from build123d import *

# Parameters (mm, degrees)
SALIENTE_EXTRUIR1_DEPTH    = 7.5
REDONDEO1_R                = 15
REDONDEO2_R                = 7.5
CORTAR_EXTRUIR1_DEPTH      = 41.485909788
CORTAR_EXTRUIR1_DEPTH_BACK = 41.485909788
CROQUIS2_R                 = 3


with BuildPart() as part:
    # Croquis1 → Saliente-Extruir1 (new, symmetric)
    with BuildSketch(Plane.XY):
        Polygon((0, 0), (-30.669872981, 0), (-30.669872981, 6), (-1.607695155, 6), (7.052558883, 11), (39.330127019, 11), (39.330127019, 5), (8.660254038, 5), align=None)
    extrude(amount=SALIENTE_EXTRUIR1_DEPTH, both=True)

    # Redondeo1
    redondeo1_edges = [part.edges().sort_by_distance(p)[0] for p in [
        (0, 0, 0),
        (-1.607695155, 6, 0),
        (7.052558883, 11, 0),
        (8.660254038, 5, 0),
    ]]
    fillet(redondeo1_edges, radius=REDONDEO1_R)

    # Redondeo2
    redondeo2_edges = [part.edges().sort_by_distance(p)[0] for p in [
        (-30.669872981, 3, -7.5),
        (-30.669872981, 3, 7.5),
        (39.330127019, 8, -7.5),
        (39.330127019, 8, 7.5),
    ]]
    fillet(redondeo2_edges, radius=REDONDEO2_R - 0.0001)  # a hair under: the kernel refuses the full size

    # Croquis2 → Cortar-Extruir1 (cut, two sides: drawn at the far end of the back side and taken through both)
    with BuildSketch(Plane(origin=(0, 6, 0), x_dir=(1, 0, 0), z_dir=(0, 1, 0)).offset(-CORTAR_EXTRUIR1_DEPTH_BACK)):
        with Locations(Location((-23.169872981, 0, 0), (0, 0, 270))):
            Circle(CROQUIS2_R)
        with Locations(Location((31.830127019, 0, 0), (0, 0, 270))):
            Circle(CROQUIS2_R)
    extrude(amount=CORTAR_EXTRUIR1_DEPTH + CORTAR_EXTRUIR1_DEPTH_BACK, mode=Mode.SUBTRACT)


solid = part.part
Work out the finished part from the listing and answer in its coordinate system (mm). A direction names the side the tool comes from. Give positions to 0.01 mm unless a question says otherwise; leave off trailing zeros. Loops run counter-clockwise (first coordinate to the right, second up) from the corner with the lowest first, then second, coordinate; pieces in that order, holes last. Notation, with made-up numbers: (4.5, -21.5) -> (39.5, -21.5) arc R16 ccw to (39.5, 2.5) -> close; hole circle Ø10 at (19.25, -26). An arc over 180 degrees is marked (long way). Use a Markdown table: item, result. Add a question column.
1) The part is cut by section A-A, the plane z = -1.5. Determine the outline of the cut face in (x, y).
2) The part is cut by section D-D, the plane x = -2. Determine the outline of the cut face in (y, z), plus the area to 3 significant figures.
3) Which of the six approach directions +Z, -Z, +X, -X, +Y, -Y give full straight-line access (tool end or side, diameter ignored) to faces 4 (the flat face through (-18, 6, 0)), 5 (the cylindrical face through (37.075, 7.958, -5.361)), 6 (the flat face through (26, 5, 0))?
4) The part is cut by section C-C, the plane z = 2. Determine the outline of the cut face in (x, y).
5) For a pull along Z with two mould halves and no side action, classify faces 1 (the cylindrical face through (-28.531, 3.042, 5.245)), 2 (the cylindrical face through (29, 8, -1)), 3 (the cylindrical face through (8.85, 4.503, 0.105)) as +Z half, -Z half, draft (parallel to the pull), parting line (faces both ways), or undercut.
6) Consider line 1 along Y through (x, z) = (30.5, 3); line 2 along Z through (x, y) = (-20.5, 5.5); line 3 along X through (y, z) = (7.45, 0). Determine where each line is inside the solid, lowest interval first.
7) Each of these flat-tipped pins is pushed along its axis until it touches: P1, Ø5, axis at y = 4, z = 5.5, coming from the -X side; P2, Ø3, axis at x = 0.5, z = 0.5, coming from the -Y side; P3, Ø4.5, axis at x = -16, z = 3, coming from the +Y side. Where does it stop, or does it pass through?
Reported:
| question | item | result |
|---|---|---|
| 1 | outline | (-30.52, 0) -> (-25.77, 0) -> (-25.77, 6) -> (-30.52, 6) -> close; (-20.57, 0) -> (-4.02, 0) arc R15 ccw to (3.48, 2.01) -> (5.18, 2.99) arc R15 cw to (12.68, 5) -> (29.23, 5) -> (29.23, 11) -> (11.07, 11) arc R15 ccw to (3.57, 8.99) -> (1.87, 8.01) arc R15 cw to (-5.63, 6) -> (-20.57, 6) -> close; (34.43, 5) -> (39.18, 5) -> (39.18, 11) -> (34.43, 11) -> close |
| 2 | outline | (0.14, -7.5) -> (6.45, -7.5) -> (6.45, 7.5) -> (0.14, 7.5) -> close |
| 2 | area | 94.6 mm^2 |
| 3 | face 4 | +Z, -Z, -X, +Y |
| 3 | face 5 | -Z, +X, +Y, -Y |
| 3 | face 6 | +Z, -Z, +X, -Y |
| 4 | outline | (-30.4, 0) -> (-25.41, 0) -> (-25.41, 6) -> (-30.4, 6) -> close; (-20.93, 0) -> (-4.02, 0) arc R15 ccw to (3.48, 2.01) -> (5.18, 2.99) arc R15 cw to (12.68, 5) -> (29.59, 5) -> (29.59, 11) -> (11.07, 11) arc R15 ccw to (3.57, 8.99) -> (1.87, 8.01) arc R15 cw to (-5.63, 6) -> (-20.93, 6) -> close; (34.07, 5) -> (39.06, 5) -> (39.06, 11) -> (34.07, 11) -> close |
| 5 | face 1 | +Z half |
| 5 | face 2 | undercut |
| 5 | face 3 | draft |
| 6 | line 1 | y = 5 to 11 |
| 6 | line 2 | z = -7.5 to -1.37, 1.37 to 7.5 |
| 6 | line 3 | x = 0.81 to 28.83, 34.83 to 39.33 |
| 7 | P1 | stops at x = -30.04 |
| 7 | P2 | stops at y = 0.31 |
| 7 | P3 | stops at y = 6 |
